Could you check a few things on this model? Use its own coordinates, in mm. A direction names the side the tool comes from. Coordinates: 2 decimals unless noted, no trailing zeros. Loops run counter-clockwise (first coordinate to the right, second up) from the corner with the lowest first, then second, coordinate; pieces in that order, holes last. Notation, with made-up numbers: M -34,-35.5 L -7,-35.5 A22 ccw -7,-15.5 Z; hole C -31,88 d7. An arc over 180 degrees is marked long. Write each question's results on one line, items separated by ' | '.
```python
from build123d import *

# Parameters (mm, degrees)
SKETCH_R        = 10
PAD_DEPTH       = 5
PAD001_DEPTH    = 5
SKETCH002_W     = 6.429408
SKETCH002_H     = 2.113688
POCKET_DEPTH    = 5
SKETCH003_R     = 2
POCKET001_DEPTH = 10.001


with BuildPart() as part:
    # Sketch → Pad (new body)
    with BuildSketch(Plane.XY):
        Circle(SKETCH_R)
    extrude(amount=PAD_DEPTH)

    # Sketch001 (on Face3 of Pad) → Pad001 (join)
    with BuildSketch(Plane.XY.offset(5)):
        Polygon((0, 8.928971), (-8.491956, 2.759204), (-5.248317, -7.223689), (5.248317, -7.223689), (8.491956, 2.759204), align=None)
    extrude(amount=PAD001_DEPTH)

    # Sketch002 (on Face2 of Pad001) → Pocket (cut)
    with BuildSketch(Plane(origin=(0, 0, 0), x_dir=(1, 0, 0), z_dir=(0, 0, -1))):
        with Locations((0, 5.755642)):
            Rectangle(SKETCH002_W, SKETCH002_H)
    extrude(amount=-POCKET_DEPTH, mode=Mode.SUBTRACT)

    # Sketch003 (on Face2 of Pocket) → Pocket001 (cut, through all)
    with BuildSketch(Plane(origin=(0, 0, 0), x_dir=(1, 0, 0), z_dir=(0, 0, -1))):
        Circle(SKETCH003_R)
    extrude(amount=-POCKET001_DEPTH, mode=Mode.SUBTRACT)


solid = part.part
```
(1) Will these pins go through, and if not, where does the flat tip stop? P1, Ø8, axis at x = 4.5, y = -1.5, coming from the -Z side; P2, Ø1.1, axis at y = -6, z = 3.5, coming from the -X side; P3, Ø6, axis at y = 4, z = 2.5, coming from the +X side; P4, Ø1.7, axis at y = -6, z = 3, coming from the +X side.
Reported:
P1: stops at z = 0 | P2: stops at x = -8.38 | P3: stops at x = 9.95 | P4: stops at x = 8.57
(2) Imagine slicing it at C-C, the plane x = 2.25. List the corners of the cut face in (y, z) for me.
Reported:
outline: M -9.74,0 L -6.81,0 L -6.81,5 L -4.7,5 L -4.7,0 L 9.74,0 L 9.74,5 L 7.29,5 L 7.29,10 L -7.22,10 L -7.22,5 L -9.74,5 Z
(3) Imagine slicing it at A-A, the plane y = 0. List the corners of the cut face in (x, z) for me.
Reported:
outline: M -10,0 L -2,0 L -2,10 L -7.6,10 L -7.6,5 L -10,5 Z; M 2,0 L 10,0 L 10,5 L 7.6,5 L 7.6,10 L 2,10 Z
(4) Which directions (+Z, -Z, +X, -X, +Y, -Y) give clear straight access to the entire face, cutting with the end or side of a thin tool? Please do faces 4 (the flat face through (0, -7.4, 5)), 5 (the flat face through (4.31, 5.8, 7.46)), 6 (the flat face through (-6.893, -2.162, 7.465)), 7 (the flat face through (3.215, -6, 2)).
Reported:
face 4: +Z | face 5: +Z, +X, +Y | face 6: +Z, -X, -Y | face 7: -Z
(5) If we mould it in two halves opening along Y, with no side actions, what happens to faces 1 (the flat face through (2, 1, 10)), 2 (the flat face through (-4.187, 5.887, 7.465)), 3 (the flat face through (0, -4.699, 2))? For each: released by +Y, released by -Y, zero draft, split by the parting line, or undercut.
Reported:
face 1: zero draft | face 2: released by +Y | face 3: undercut
(6) Imagine slicing it at B-B, the plane z = 5.5. List the corners of the cut face in (x, y) for me.
Reported:
outline: M -8.49,2.76 L -5.25,-7.22 L 5.25,-7.22 L 8.49,2.76 L 0,8.93 Z; hole C 0,0 d4
(7) Please list where these lines run through material, in increasing order: probe 1 along Y at (x, z) = (0, 4.25); probe 2 along Z at (x, y) = (-5.5, -7.25); probe 3 along X at (y, z) = (0, 5.25). Write a range as from..to.
Reported:
probe 1: y = -10..-6.81, -4.7..-2, 2..10 | probe 2: z = 0..5 | probe 3: x = -7.6..-2, 2..7.6
(8) Imagine slicing it at D-D, the plane z = 1.25. List the corners of the cut face in (x, y) for me, and give its area (3 significant figures).
Reported:
outline: C 0,0 d20; hole M -3.21,-6.81 L 3.21,-6.81 L 3.21,-4.7 L -3.21,-4.7 Z; hole C 0,0 d4 | area: 288 mm2
